Design review of the part shown in the three views and the two pictorial views. Dimensions are in mm from the part's minimum x, y and z. A direction names the side the tool comes from. Round coordinates to 2 decimals unless told otherwise and drop trailing zeros. Order: outer loops, then holes, each group sorted by start corner. A loop starts at its lowest first (then second) coordinate and runs counter-clockwise, first axis right, second up. Notation, with made-up numbers: (14.5, -20.75) - (54.5, -20.75) arc R16 ccw to (54.5, 10.25) - close; hole circle Ø7 at (31, -26.75). An arc over 180 degrees is marked (long way). One line per item, written item: value.
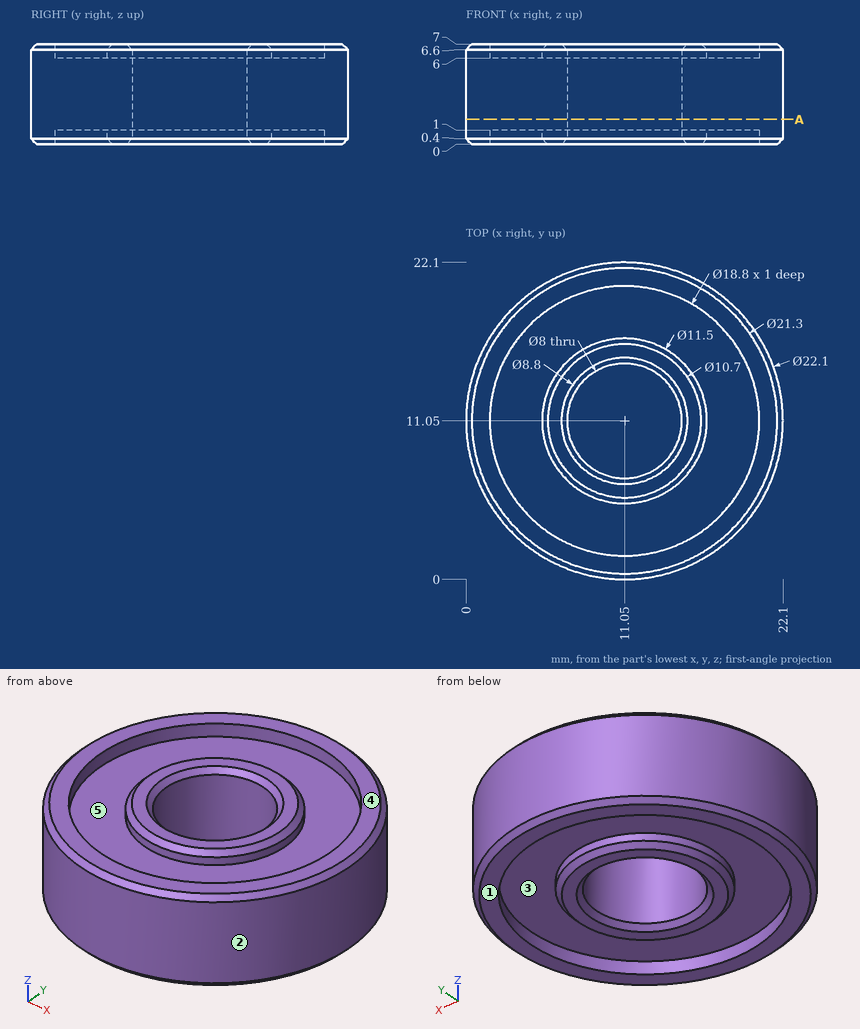
Item 1: The part is to be moulded in two halves that separate along X. For the marked faces 1, 2 and 3, say which applies: +X half, -X half, draft (parallel to the pull), parting line (faces both ways), or undercut.
Returned:
face 1: draft
face 2: parting line
face 3: undercut
Item 2: Wall thickness on line 1 (Y direction, x = 11.05, z = 6.3); line 2 (X direction, y = 11, z = 5.5): over which ranges is each line inside the solid? List them lowest first.
Returned:
line 1: 0 to 1.65, 5.3 to 7.05, 15.05 to 16.8, 20.45 to 22.1
line 2: 0 to 7.05, 15.05 to 22.1
Item 3: Take a section at A-A (z = 1.75). Write out the cut boundary in (x, y), plus the area to 3 significant figures.
Returned:
outline: circle Ø22.1 at (11.05, 11.05); hole circle Ø8 at (11.05, 11.05)
area: 333 mm^2
Item 4: Machinability: for the marked faces 4 and 5, which of the approach directions +Z, -Z, +X, -X, +Y, -Y give a long, thin tool a straight path to every point of the face, cutting with its end or side? Answer none if there is none.
Returned:
face 4: +Z, +X, -X, +Y, -Y
face 5: +Z
Item 5: For P1, Ø7, axis at x = 11.05, y = 11.05, coming from the -Z side; P2, Ø2, axis at x = 14.5, y = 4.5, coming from the +Z side; P3, Ø5.5, axis at x = 12, y = 10, coming from the +Z side; P4, Ø1, axis at x = 15, z = 5, coming from the -Y side, all flat-tipped, find the tip position at first contact; note any pin that passes through.
Returned:
P1: through
P2: z = 6
P3: z = 6.77
P4: y = 0.55
